from build123d import *

# Parameters (mm, degrees)
F0_W     = 98
F0_H     = 32
F1_DEPTH = 19.05


with BuildPart() as f1:
    # F0 (on Top) → F1 (new body)
    with BuildSketch(Plane.XY):
        with BuildLine():
            Line((276.225, -127), (292.1, -127))
            ThreePointArc((292.1, -127), (310.060512, -119.560512), (317.5, -101.6))
            Line((317.5, -101.6), (317.5, 101.6))
            ThreePointArc((317.5, 101.6), (310.060512, 119.560512), (292.1, 127))
            Line((292.1, 127), (-292.1, 127))
            ThreePointArc((-292.1, 127), (-310.060512, 119.560512), (-317.5, 101.6))
            Line((-317.5, 101.6), (-317.5, -101.6))
            ThreePointArc((-317.5, -101.6), (-310.060512, -119.560512), (-292.1, -127))
            Line((-292.1, -127), (69.85, -127))
            Line((69.85, -127), (69.85, -107.95))
            ThreePointArc((69.85, -107.95), (54.134552, -101.440448), (47.625, -85.725))
            Line((47.625, -85.725), (47.625, 80.9625))
            ThreePointArc((47.625, 80.9625), (54.134552, 96.677948), (69.85, 103.1875))
            Line((69.85, 103.1875), (276.225, 103.1875))
            ThreePointArc((276.225, 103.1875), (291.940448, 96.677948), (298.45, 80.9625))
            Line((298.45, 80.9625), (298.45, -85.725))
            ThreePointArc((298.45, -85.725), (291.940448, -101.440448), (276.225, -107.95))
            Line((276.225, -107.95), (276.225, -127))
        make_face()
        with Locations((-49, 87.1875)):
            Rectangle(F0_W, F0_H, mode=Mode.SUBTRACT)
        with BuildLine():
            Line((276.225, -97.762614), (276.225, -107.95))
            ThreePointArc((276.225, -107.95), (291.940448, -101.440448), (298.45, -85.725))
            Line((298.45, -85.725), (298.45, 80.9625))
            ThreePointArc((298.45, 80.9625), (291.940448, 96.677948), (276.225, 103.1875))
            Line((276.225, 103.1875), (69.85, 103.1875))
            ThreePointArc((69.85, 103.1875), (54.134552, 96.677948), (47.625, 80.9625))
            Line((47.625, 80.9625), (47.625, -85.725))
            ThreePointArc((47.625, -85.725), (54.134552, -101.440448), (69.85, -107.95))
            Line((69.85, -107.95), (69.85, -97.762614))
            Line((69.85, -97.762614), (276.225, -97.762614))
        make_face()
    extrude(amount=F1_DEPTH)


solid = f1.part
Read the model definition and answer for the solid it produces. Units are mm, in the model's axes. A direction names the side the tool comes from. Coordinates: 2 decimals unless noted, no trailing zeros. Write each loop counter-clockwise with the first axis right and the second up, starting at its lowest first coordinate (ties: lowest second). Pieces come first, ordered by that corner, then holes. Notation, with made-up numbers: (26.5, 86) -> (47.5, 86) arc R27 cw to (47.5, 106) -> close; hole circle Ø3 at (1, -14.75). An arc over 180 degrees is marked (long way). Return JSON: item names as keys, results as strings.
(1) The part is cut by section C-C on x = 233. Give the vertices of the cut face in (y, z), then the cut area to 3 significant figures.
Answers below:
{"outline": "(-97.76, 0) -> (127, 0) -> (127, 19.05) -> (-97.76, 19.05) -> close", "area": "4,280 mm^2"}
(2) The part is cut by section A-A on x = -8.5. Give the vertices of the cut face in (y, z), then the cut area to 3 significant figures.
Answers below:
{"outline": "(-127, 0) -> (71.19, 0) -> (71.19, 19.05) -> (-127, 19.05) -> close; (103.19, 0) -> (127, 0) -> (127, 19.05) -> (103.19, 19.05) -> close", "area": "4,230 mm^2"}
(3) Each of these flat-tipped pins is pushed along its axis until it touches: P1, Ø1.5, axis at x = 164, z = 11, coming from the -Y side; P2, Ø5.5, axis at y = -118.5, z = 12, coming from the +X side. Where does it stop, or does it pass through?
Answers below:
{"P1": "y = -97.76", "P2": "x = 313.19"}
(4) Consider line 1 along Y through (x, z) = (-16, 7.5); line 2 along Y through (x, z) = (139.5, 11); line 3 along X through (y, z) = (113, 14). Determine where each line is inside the solid, lowest interval first. Write a range as from..to.
Answers below:
{"line 1": "-127..71.19, 103.19..127", "line 2": "-97.76..127", "line 3": "-314.8..314.8"}
(5) For a pull along X with two mould halves and no side action, classify faces 1 (the cylindrical face through (-310.26, -119.36, 9.39)), 2 (the flat face through (276.225, -112, 9)), 3 (the flat face through (284, -127, 9)), 4 (the flat face through (-50, 103.188, 9)) as pulls with the +X half, pulls with the -X half, needs draft (parallel to the pull), parting line crosses it, or undercut.
Answers below:
{"face 1": "pulls with the -X half", "face 2": "undercut", "face 3": "needs draft", "face 4": "undercut"}
(6) Which of the six approach directions +Z, -Z, +X, -X, +Y, -Y give full straight-line access (tool end or side, diameter ignored) to faces 5 (the flat face through (-50, 71.188, 9)), 6 (the flat face through (172, -97.763, 9)), 7 (the cylindrical face through (-309.86, 119.76, 9.39))?
Answers below:
{"face 5": "+Z, -Z", "face 6": "+Z, -Z, -Y", "face 7": "+Z, -Z, -X, +Y"}
